from build123d import *

# Parameters (mm, degrees)
SKETCH_1_W          = 47
SKETCH_1_H          = 65
EXTRUDE_1_DEPTH     = 17
CUT_EXTRUDE_1_DEPTH = 59
CUT_EXTRUDE_2_DEPTH = 79.571641677
EXTRUDE_2_DEPTH     = 10
SKETCH_7_R          = 4.2
CUT_EXTRUDE_3_DEPTH = 10
SKETCH_8_R          = 2.25
CUT_EXTRUDE_4_DEPTH = 79.571641677
CUT_EXTRUDE_5_DEPTH = 10
CUT_EXTRUDE_START   = -10
SKETCH_10_R         = 12.5
SKETCH_10_R_2       = 10
CUT_EXTRUDE_6_DEPTH = 6
CUT_EXTRUDE_START_2 = -20
SKETCH_11_R         = 12.5
SKETCH_11_R_2       = 10
CUT_EXTRUDE_7_DEPTH = 6


with BuildPart() as part:
    # Эскиз1 → Бобышка-Вытянуть1 (new body)
    with BuildSketch(Plane(origin=(0, 0, 0), x_dir=(1, 0, 0), z_dir=(0, 1, 0))):
        with Locations((-17.236996401, 32.5)):
            Rectangle(SKETCH_1_W, SKETCH_1_H)
    extrude(amount=EXTRUDE_1_DEPTH)

    # Эскиз2 → Вырез-Вытянуть1 (cut)
    with BuildSketch(Plane.XY.offset(-3)):
        with BuildLine():
            Line((-22.486996401, 7.5), (-22.486996401, 0))
            Line((-22.486996401, 0), (-40.736996401, 0))
            Line((-40.736996401, 0), (-40.736996401, 7.5))
            Line((-40.736996401, 7.5), (-37.986996401, 7.5))
            ThreePointArc((-37.986996401, 7.5), (-30.236996401, 15.25), (-22.486996401, 7.5))
        make_face()
    extrude(amount=-CUT_EXTRUDE_1_DEPTH, mode=Mode.SUBTRACT)

    # Эскиз5 → Вырез-Вытянуть2 (cut, through all)
    with BuildSketch(Plane.XY):
        with BuildLine():
            Line((-35.986996401, 7.5), (-40.736996401, 7.5))
            Line((-40.736996401, 7.5), (-40.736996401, 0))
            Line((-40.736996401, 0), (-24.486996401, 0))
            Line((-24.486996401, 0), (-24.486996401, 7.5))
            ThreePointArc((-24.486996401, 7.5), (-30.236996401, 13.25), (-35.986996401, 7.5))
        make_face()
    extrude(amount=-CUT_EXTRUDE_2_DEPTH, mode=Mode.SUBTRACT)

    # Эскиз6 → Бобышка-Вытянуть2 (add)
    with BuildSketch(Plane.XY.offset(-27.5)):
        with BuildLine():
            Line((-35.986996401, 7.5), (-40.736996401, 7.5))
            Line((-40.736996401, 7.5), (-40.736996401, 17))
            Line((-40.736996401, 17), (-24.486996401, 17))
            Line((-24.486996401, 17), (-22.486996401, 17))
            Line((-22.486996401, 17), (-22.486996401, 0))
            Line((-22.486996401, 0), (-24.486996401, 0))
            Line((-24.486996401, 0), (-24.486996401, 7.5))
            ThreePointArc((-24.486996401, 7.5), (-30.236996401, 13.25), (-35.986996401, 7.5))
        make_face()
    extrude(amount=-EXTRUDE_2_DEPTH)

    # Эскиз7 → Вырез-Вытянуть3 (cut)
    with BuildSketch(Plane(origin=(6.263003599, 0, 0), x_dir=(0, 0, -1), z_dir=(1, 0, 0))):
        with Locations((8.125, 8.5)):
            Circle(SKETCH_7_R)
        with Locations((56.875, 8.5)):
            Circle(SKETCH_7_R)
    extrude(amount=-CUT_EXTRUDE_3_DEPTH, mode=Mode.SUBTRACT)

    # Эскиз8 → Вырез-Вытянуть4 (cut, through all)
    with BuildSketch(Plane(origin=(0, 17, 0), x_dir=(1, 0, 0), z_dir=(0, 1, 0))):
        with Locations(Location((-8.736996401, 8.125, 0), (0, 0, 270))):
            Circle(SKETCH_8_R)
        with Locations(Location((-8.736996401, 56.875, 0), (0, 0, 270))):
            Circle(SKETCH_8_R)
    extrude(amount=-CUT_EXTRUDE_4_DEPTH, mode=Mode.SUBTRACT)

    # Эскиз9 → Вырез-Вытянуть5 (cut)
    with BuildSketch(Plane.XZ):
        Polygon((-4.406869382, -56.875), (-6.571932892, -53.125), (-10.902059911, -53.125), (-13.06712342, -56.875), (-10.902059911, -60.625), (-6.571932892, -60.625), align=None)
        Polygon((-4.406869382, -8.125), (-6.571932892, -4.375), (-10.902059911, -4.375), (-13.06712342, -8.125), (-10.902059911, -11.875), (-6.571932892, -11.875), align=None)
    extrude(amount=-CUT_EXTRUDE_5_DEPTH, mode=Mode.SUBTRACT)

    # Эскиз10 → Вырез-Вытянуть6 (cut)
    with BuildSketch(Plane.XY.offset(-3).offset(CUT_EXTRUDE_START)):
        with Locations((-30.236996401, 7.5)):
            Circle(SKETCH_10_R)
        with Locations((-30.236996401, 7.5)):
            Circle(SKETCH_10_R_2, mode=Mode.SUBTRACT)
    extrude(amount=-CUT_EXTRUDE_6_DEPTH, mode=Mode.SUBTRACT)

    # Эскиз11 → Вырез-Вытянуть7 (cut)
    with BuildSketch(Plane.XY.offset(-27.5).offset(CUT_EXTRUDE_START_2)):
        with Locations((-30.236996401, 7.5)):
            Circle(SKETCH_11_R)
        with Locations((-30.236996401, 7.5)):
            Circle(SKETCH_11_R_2, mode=Mode.SUBTRACT)
    extrude(amount=-CUT_EXTRUDE_7_DEPTH, mode=Mode.SUBTRACT)


solid = part.part
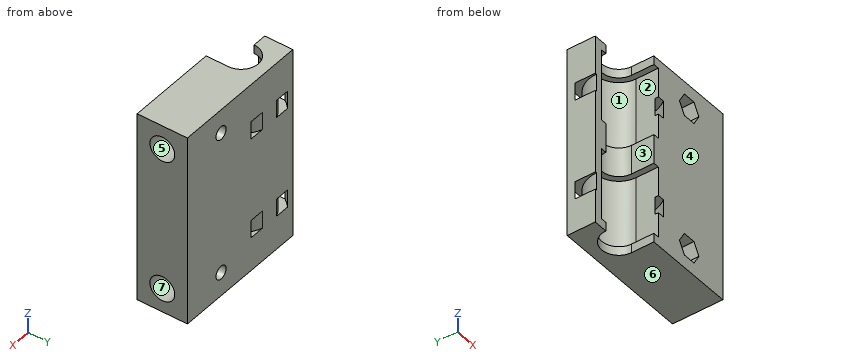
CAD build for the part. Positions are in the model's coordinates, mm. Face numbers are marked on the shaded views. A direction names the side the tool comes from. Round coordinates to 2 decimals unless told otherwise and drop trailing zeros. Write each loop counter-clockwise with the first axis right and the second up, starting at its lowest first coordinate (ties: lowest second). Pieces come first, ordered by that corner, then holes.
(1) Drop flat-ended pins along their axis: P1, Ø0.9, axis at y = 4.5, z = -1, coming from the -X side; P2, Ø4.5, axis at x = -33, y = 9, coming from the +Z side; P3, Ø8, axis at y = 5, z = -50, coming from the -X side; P4, Ø6, axis at y = 3.5, z = -45.5, coming from the -X side. Give the stop position or say it passes through.
(2) Slice it at D-D, the plane y = 8.5. Count the separate pieces of the cut face and the enclosed holes in it, and give its area (3 significant figures).
(3) 3-axis set-ups, long thin cutter, end or side, ignore diameter. For the marked faces 1, 2 and 3: which of +Z, -Z, +X, -X, +Y, -Y reach the whole face in a straight line?
(4) Slice it at C-C, the plane x = 0. Write the cut outline in (y, z) (3 decimals), and give its area (3 significant figures).
(5) Probe line 1 along Z through (x, y) = (-10, 4.25) (3 decimals); line 2 along X through (y, z) = (8, -48); line 3 along Z through (x, y) = (-24.5, 10.5). List the from-to ranges inside material, lowest first.
(6) Slice it at B-B, the plane z = -26. Write the cut outline in (x, y), and give its area (3 significant figures).
(7) Slice it at A-A, the plane z = -16. Write the cut outline in (x, y), and give its area (3 significant figures).
(8) Mould opens along Y. For the marked faces 4, 5, 6 and 7 say: pulls with the +Y half, pulls with the -Y half, needs draft (parallel to the pull), parting line crosses it, or undercut.
From the geometry:
1. P1: stops at x = -24.49
1. P2: passes through
1. P3: stops at x = -40.74
1. P4: stops at x = -22.49
2. separate pieces: 2
2. enclosed holes: 4
2. area: 1,820 mm2
3. face 1: -Y
3. face 2: -X, -Y
3. face 3: +Z, -Z, -X, -Y
4. outline: (0, -65) - (17, -65) - (17, 0) - (0, 0) - close; hole circle Ø8.4 at (8.5, -56.875); hole circle Ø8.4 at (8.5, -8.125)
4. area: 994 mm2
5. line 1: z = -65 to -60.625, -53.125 to -11.875, -4.375 to 0
5. line 2: x = -40.22 to -37.97, -22.5 to -20.25, -17.75 to 6.26
5. line 3: z = -65 to -62, -37.5 to -27.5, -3 to 0
6. outline: (-40.74, 7.5) - (-37.99, 7.5) arc R7.75 cw to (-22.49, 7.5) - (-22.49, 0) - (6.26, 0) - (6.26, 17) - (-40.74, 17) - close
6. area: 568 mm2
7. outline: (-40.74, 14.28) arc R12.5 cw to (-38.36, 17) - (-40.74, 17) - close; (-40.24, 7.5) - (-37.99, 7.5) arc R7.75 cw to (-22.49, 7.5) - (-22.49, 1.18) arc R10 ccw to (-27.11, 17) - (-33.36, 17) arc R10 ccw to start; (-22.11, 17) arc R12.5 cw to (-20.24, 0) - (6.26, 0) - (6.26, 17) - close
7. area: 500 mm2
8. face 4: pulls with the -Y half
8. face 5: undercut
8. face 6: needs draft
8. face 7: undercut
